Autodesk Fusion 360 part; units mm, degrees
sketch "Sketch1" plane through (0, 0, 0) normal (0, 1, 0) x (1, 0, 0)
  line L0 (0, 0) -> (-15, 0)
  line L1 (-15, 0) -> (-15, -6)
  line L2 (-15, -6) -> (-20, -6)
  line L3 (-20, -6) -> (-20, 0)
  line L4 (-20, 0) -> (-25, 0)
  line L5 (-7.5, 20) -> (0, 20)
  line L6 (0, 0) -> (15, 0)
  line L7 (15, 0) -> (15, -6)
  line L8 (15, -6) -> (20, -6)
  line L9 (20, -6) -> (20, 0)
  line L10 (20, 0) -> (25, 0)
  line L11 (7.5, 20) -> (0, 20)
  line L12 (-25, 0) -> (-11.5, 18)
  line L13 (25, 0) -> (11.5, 18)
  arc A0 (-7.5, 20) -> (-11.5, 18) centre (-7.5, 15) ccw
  arc A1 (11.5, 18) -> (7.5, 20) centre (7.5, 15) ccw
  line L14 (0, 13) -> (-4.5, 13)
  line L15 (-4.5, 13) -> (-4.5, 7.5)
  line L16 (-4.5, 7.5) -> (4.5, 7.5)
  line L17 (0, 13) -> (4.5, 13)
  line L18 (4.5, 13) -> (4.5, 7.5)
  circle A2 centre (0, 2.5) radius 1.5
  dimension "d1" = 5
  dimension "d6" = 2.5
  dimension "d7" = 3
extrude "Extrude1" add sketch "Sketch1" along normal blind 5
sketch "Sketch2" plane through (0, 5, 0) normal (0, 1, 0) x (-1, 0, 0)
  line L0 (4.5, -13) -> (-4.5, -13)
  line L1 (-4.5, -13) -> (-4.5, -7.5)
  line L2 (-4.5, -7.5) -> (4.5, -7.5)
  line L3 (4.5, -7.5) -> (4.5, -13)
  circle A0 centre (0, -2.5) radius 1.5
  line L4 (15, 0) -> (-15, 0)
  line L5 (-15, 0) -> (-15, 6)
  line L6 (-15, 6) -> (-20, 6)
  line L7 (-20, 6) -> (-20, 0)
  line L8 (-20, 0) -> (-25, 0)
  line L9 (-25, 0) -> (-11.5, -18)
  arc A1 (-11.5, -18) -> (-7.5, -20) centre (-7.5, -15) ccw
  line L10 (-7.5, -20) -> (7.5, -20)
  arc A2 (7.5, -20) -> (11.5, -18) centre (7.5, -15) ccw
  line L11 (11.5, -18) -> (25, 0)
  line L12 (25, 0) -> (20, 0)
  line L13 (20, 0) -> (20, 6)
  line L14 (20, 6) -> (15, 6)
  line L15 (15, 6) -> (15, 0)
fillet "Fillet1" radius 2 5 edges at (18.25, 5, -9) (9.7361, 5, -19.4721) (0, 5, -20) (-9.7361, 5, -19.4721) (-18.25, 5, -9)
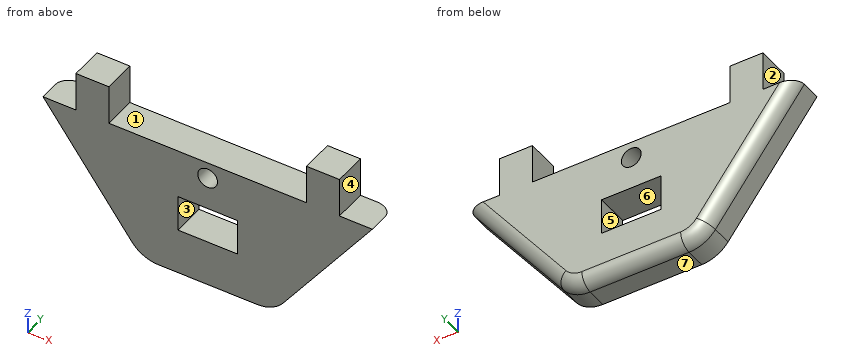
Here's how the part is built. I have some questions about the finished solid (model axes, mm). Face numbers are marked on the shaded views. A direction names the side the tool comes from. Round coordinates to 2 decimals unless told otherwise and drop trailing zeros. Write each loop counter-clockwise with the first axis right and the second up, starting at its lowest first coordinate (ties: lowest second). Pieces come first, ordered by that corner, then holes.
1. I need wall thicknesses on L1, parallel to Z at x = 0, y = 2.75; L2, parallel to Z at x = 2.5, y = 1.2; L3, parallel to X at y = 3.6, z = -2.5. Which ranges of each line are inside material? Lowest first, please.
2. If we mould it in two halves opening along Z, with no side actions, what happens to the marked faces 4, 5, 6 and 7? For each: released by +Z, released by -Z, zero draft, split by the parting line, or undercut.
3. Suppose I cut it at A-A (z = 1.5). List the corners of the cut face in (x, y) for me.
4. For the marked faces 1, 2 and 3, which set-ups out of +Z, -Z, +X, -X, +Y, -Y let a thin tool reach every point of the face, with its end or its side?
5. Suppose I cut it at C-C (x = 0). List the corners of the cut face in (y, z) for me.
6. Suppose I cut it at B-B (y = 1.25). List the corners of the cut face in (x, z) for me, and give its area (3 significant figures).
7. Suppose I cut it at D-D (x = 5). List the corners of the cut face in (y, z) for me.
8. Will these pins go through, and if not, where does the flat tip stop? pin 1 Ø2 at (y, z) = (3.5, -10) entering from +X; pin 2 Ø1.5 at (x, y) = (-6, 2.5) entering from +Z; pin 3 Ø2.5 at (y, z) = (3.5, -11.5) entering from -X.
Answer sheet:
1. L1: z = -20 to -13, -7.5 to -4, -1 to 0
1. L2: z = -20 to -13, -7.5 to 0
1. L3: x = -23.01 to -1.5, 1.5 to 23.01
2. face 4: zero draft
2. face 5: undercut
2. face 6: undercut
2. face 7: released by -Z
3. outline: (-20, 0) - (-15, 0) - (-15, 5) - (-20, 5) - close; (15, 0) - (20, 0) - (20, 5) - (15, 5) - close
4. face 1: +Z, +Y, -Y
4. face 2: +Z, -X, +Y, -Y
4. face 3: +Y, -Y
5. outline: (0, -20) - (3, -20) arc R2 ccw to (5, -18) - (5, -13) - (0, -13) - close; (0, -7.5) - (5, -7.5) - (5, -4) - (0, -4) - close; (0, -1) - (5, -1) - (5, 0) - (0, 0) - close
6. outline: (-25, 0) - (-11.5, -18) arc R5 ccw to (-7.5, -20) - (7.5, -20) arc R5 ccw to (11.5, -18) - (25, 0) - (20, 0) - (20, 6) - (15, 6) - (15, 0) - (-15, 0) - (-15, 6) - (-20, 6) - (-20, 0) - close; hole (-4.5, -13) - (4.5, -13) - (4.5, -7.5) - (-4.5, -7.5) - close; hole circle Ø3 at (0, -2.5)
6. area: 702 mm2
7. outline: (0, -20) - (3, -20) arc R2 ccw to (5, -18) - (5, 0) - (0, 0) - close
8. pin 1: stops at x = 18.21
8. pin 2: stops at z = 0
8. pin 3: stops at x = -17.27
